Part model, mm, in its own coordinate system. A direction names the side the tool comes from. Coordinates: 2 decimals unless noted, no trailing zeros. Loops run counter-clockwise (first coordinate to the right, second up) from the corner with the lowest first, then second, coordinate; pieces in that order, holes last. Notation, with made-up numbers: (12.25, 48) -> (56.25, 48) arc R27 ccw to (56.25, 85) -> close; hole circle Ø10 at (60.5, 54). An arc over 180 degrees is marked (long way). One line per question, with ' | ' between items. Start each with the question number.
1) Drop flat-ended pins along their axis: pin 1 (1.5 mm diameter, centred on x = -131.5, z = 27.5, fed in from +Y); pin 2 (1 mm diameter, centred on y = -28.5, z = 16.5, fed in from -X); pin 3 (1.5 mm diameter, centred on y = 39, z = -12.5, fed in from -X). Give the stop position or say it passes through.
2) Cut at D-D (y = 32.5). List the corners of the cut face in (x, z).
3) Two-plate mould, pull along Y, no slides. Class faces 3 (the face through (-82, -29.624, 1)), 4 (the face through (-98, -27.624, 1)), 5 (the face through (-139.633, -28.61, -34.773)), 6 (the face through (-30.99, 3.23, -59.57)): released by +Y, released by -Y, zero draft, split by the parting line, or undercut.
4) Cut at C-C (z = 29.5). List the corners of the cut face in (x, y), plus the area to 3 significant figures.
5) Probe L1, parallel to Z at x = -160.5, y = -28.9; L2, parallel to Z at x = -91.65, y = -29.2; L3, parallel to Y at x = -124, z = -15. List the from-to ranges inside material, lowest first. Write a range as from..to.
6) Cut at A-A (x = -137.65). List the corners of the cut face in (y, z).
7) Cut at B-B (z = -0.5). List the corners of the cut face in (x, y).
8) 3-axis set-ups, long thin cutter, end or side, ignore diameter. For faces 1 (the face through (-32, 22, 1)), 2 (the face through (-62, -28, 63.696)): which of +Z, -Z, +X, -X, +Y, -Y reach the whole face in a straight line?
from build123d import *

# Parameters (mm, degrees)
SKETCH_1_W          = 127.39196645
SKETCH_1_H          = 99.499845157
SKETCH_1_R          = 2
EXTRUDE_1_DEPTH     = 2
SKETCH_2_W          = 127.39196645
SKETCH_2_H          = 2
EXTRUDE_2_DEPTH     = 115.4
SKETCH_4_R          = 2
CUT_EXTRUDE_1_DEPTH = 144.079097981
SKETCH_6_R          = 3.5
CUT_EXTRUDE_2_DEPTH = 166.366738145
SKETCH_7_R          = 3
EXTRUDE_3_DEPTH     = 2
FILLET_1_R          = 5
SKETCH_8_W          = 161.877108061
SKETCH_8_H          = 133.071465469
CUT_EXTRUDE_3_DEPTH = 179.583476668


with BuildPart() as part:
    # Эскиз1 → Бобышка-Вытянуть1 (new body)
    with BuildSketch(Plane(origin=(0, 0, 0), x_dir=(0, 0, -1), z_dir=(1, 0, 0))):
        with Locations((0, 20.12589484)):
            Rectangle(SKETCH_1_W, SKETCH_1_H)
        with Locations((11.663084527, 42.625972261)):
            Circle(SKETCH_1_R, mode=Mode.SUBTRACT)
        with Locations((57.663084527, 42.625972261)):
            Circle(SKETCH_1_R, mode=Mode.SUBTRACT)
        with Locations((57.663084527, 2.625972261)):
            Circle(SKETCH_1_R, mode=Mode.SUBTRACT)
        with Locations((11.663084527, 2.625972261)):
            Circle(SKETCH_1_R, mode=Mode.SUBTRACT)
        with Locations(Location((-11.836915473, 2.625972261, 0), (0, 0, 180))):
            Circle(SKETCH_1_R, mode=Mode.SUBTRACT)
        with Locations(Location((-57.836915473, 2.625972261, 0), (0, 0, 180))):
            Circle(SKETCH_1_R, mode=Mode.SUBTRACT)
        with Locations(Location((-57.836915473, 42.625972261, 0), (0, 0, 180))):
            Circle(SKETCH_1_R, mode=Mode.SUBTRACT)
        with Locations(Location((-11.836915473, 42.625972261, 0), (0, 0, 180))):
            Circle(SKETCH_1_R, mode=Mode.SUBTRACT)
    extrude(amount=EXTRUDE_1_DEPTH)

    # Эскиз2 → Бобышка-Вытянуть2 (add)
    with BuildSketch(Plane(origin=(2, 0, 0), x_dir=(0, 0, -1), z_dir=(1, 0, 0))):
        with Locations((0, -28.624027739)):
            Rectangle(SKETCH_2_W, SKETCH_2_H)
    extrude(amount=EXTRUDE_2_DEPTH)

    # Эскиз4 → Вырез-Вытянуть1 (cut, through all)
    with BuildSketch(Plane(origin=(0, 21.675972261, 0), x_dir=(1, 0, 0), z_dir=(0, 1, 0))):
        with Locations(Location((61.65, 34.512555998, 0), (0, 0, 270))):
            Circle(SKETCH_4_R)
        with Locations(Location((61.65, -5.487444002, 0), (0, 0, 270))):
            Circle(SKETCH_4_R)
        with Locations(Location((107.65, -5.487444002, 0), (0, 0, 270))):
            Circle(SKETCH_4_R)
        with Locations(Location((107.65, 34.512555998, 0), (0, 0, 270))):
            Circle(SKETCH_4_R)
    extrude(amount=-CUT_EXTRUDE_1_DEPTH, mode=Mode.SUBTRACT)

    # Эскиз6 → Вырез-Вытянуть2 (cut, through all)
    with BuildSketch(Plane(origin=(0, -27.624027739, 0), x_dir=(1, 0, 0), z_dir=(0, 1, 0))):
        with Locations(Location((62.669967975, -49.504016775, 0), (0, 0, 270))):
            Circle(SKETCH_6_R)
        with Locations(Location((40.99052879, -0.086168012, 0), (0, 0, 270))):
            Circle(SKETCH_6_R)
    extrude(amount=-CUT_EXTRUDE_2_DEPTH, mode=Mode.SUBTRACT)

    # Эскиз7 → Бобышка-Вытянуть3 (add)
    with BuildSketch(Plane(origin=(0, -27.624027739, 0), x_dir=(1, 0, 0), z_dir=(0, 1, 0))):
        with BuildLine():
            Line((130.5, 51.195983225), (117.4, 51.195983225))
            Line((117.4, 51.195983225), (117.4, 63.195983225))
            Line((117.4, 63.195983225), (130.5, 63.195983225))
            ThreePointArc((130.5, 63.195983225), (136.5, 57.195983225), (130.5, 51.195983225))
        make_face()
        with Locations(Location((130.5, 57.195983225, 0), (0, 0, 270))):
            Circle(SKETCH_7_R, mode=Mode.SUBTRACT)
    extrude(amount=-EXTRUDE_3_DEPTH)

    # Скругление1
    fillet_1_edges = [part.edges().sort_by_distance(p)[0] for p in [
        (117.4, -28.624027739, -51.195983225),
    ]]
    fillet(fillet_1_edges, radius=FILLET_1_R)


with BuildPart() as body_2:
    # Зеркальное отражение1: mirrored copy
    add(part.part.mirror(Plane.ZY.offset(15)))


with BuildPart() as part_1:
    add(part.part)

    # Эскиз8 → Вырез-Вытянуть3 (cut, through all)
    with BuildSketch(Plane.ZY.offset(15)):
        with Locations((1.413773869, 20.567699173)):
            Rectangle(SKETCH_8_W, SKETCH_8_H)
    extrude(amount=-CUT_EXTRUDE_3_DEPTH, mode=Mode.SUBTRACT)


solid = body_2.part
Reported:
1) pin 1: stops at y = -27.62 | pin 2: stops at x = -147.4 | pin 3: stops at x = -32
2) outline: (-32, -63.7) -> (-30, -63.7) -> (-30, 63.7) -> (-32, 63.7) -> close
3) face 3: released by -Y | face 4: released by +Y | face 5: zero draft | face 6: undercut
4) outline: (-147.4, -29.62) -> (-30, -29.62) -> (-30, 69.88) -> (-32, 69.88) -> (-32, -27.62) -> (-147.4, -27.62) -> close | area: 430 mm²
5) L1: z = -63.2..-60.2, -54.2..-51.2 | L2: z = -63.7..-36.51, -32.51..3.49, 7.49..46.16, 52.85..63.7 | L3: y = -29.62..-27.62
6) outline: (-29.62, -63.7) -> (-27.62, -63.7) -> (-27.62, -36.51) -> (-29.62, -36.51) -> close; (-29.62, -32.51) -> (-27.62, -32.51) -> (-27.62, 3.49) -> (-29.62, 3.49) -> close; (-29.62, 7.49) -> (-27.62, 7.49) -> (-27.62, 63.7) -> (-29.62, 63.7) -> close
7) outline: (-147.4, -29.62) -> (-74.44, -29.62) -> (-74.44, -27.62) -> (-147.4, -27.62) -> close; (-67.54, -29.62) -> (-30, -29.62) -> (-30, 69.88) -> (-32, 69.88) -> (-32, -27.62) -> (-67.54, -27.62) -> close
8) face 1: +Z, -Z, -X, +Y | face 2: +Z, +X, -X, +Y, -Y
